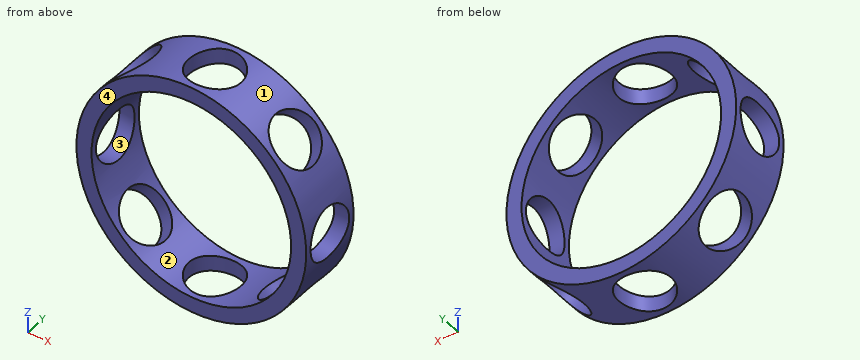
```python
from build123d import *

# Parameters (mm, degrees)
BOSS_EXTRUDE1_DEPTH      = 0.93218
BOSS_EXTRUDE1_DEPTH_BACK = 0.93218
SKETCH1_R                = 3.39852
SKETCH1_R_2              = 2.95148
CUT_EXTRUDE1_REACH       = 6.896
CUT_EXTRUDE1_END_RADIUS  = 3.39852
SKETCH3_R                = 0.762
CIRPATTERN1_COUNT        = 8


with BuildPart() as part:
    # Sketch1 → Boss-Extrude1 (new, two sides: drawn at the far end of the back side and taken through both)
    with BuildSketch(Plane(origin=(0, 0, 0), x_dir=(1, 0, 0), z_dir=(0, 1, 0)).offset(-BOSS_EXTRUDE1_DEPTH_BACK)):
        with Locations(Location((0, 0, 0), (0, 0, 270))):
            Circle(SKETCH1_R)
        with Locations(Location((0, 0, 0), (0, 0, 270))):
            Circle(SKETCH1_R_2, mode=Mode.SUBTRACT)
    extrude(amount=BOSS_EXTRUDE1_DEPTH + BOSS_EXTRUDE1_DEPTH_BACK)

    # Cut-Extrude1: up to this cylinder (the profile starts inside it)
    cut_extrude1_end = Plane(origin=(0, 0, 0), z_dir=(0, 1, 0)) * Cylinder(CUT_EXTRUDE1_END_RADIUS, 21.58904, mode=Mode.PRIVATE)
    # Sketch3 → Cut-Extrude1 (cut, up to the surface)
    with BuildSketch(Plane.XY, mode=Mode.PRIVATE) as cut_extrude1_sk1:
        Circle(SKETCH3_R)
    cut_extrude1_tool1 = extrude(cut_extrude1_sk1.sketch, amount=-CUT_EXTRUDE1_REACH, mode=Mode.PRIVATE) & cut_extrude1_end
    cut_extrude1 = cut_extrude1_tool1.solids().sort_by_distance((0, 0, 0))[0]
    add(cut_extrude1, mode=Mode.SUBTRACT)

    # CirPattern1: Cut-Extrude1 ×8 about axis
    cirpattern1_axis = Axis((0, 0, 0), (0, 1, 0))
    for i in range(1, CIRPATTERN1_COUNT):
        add(cut_extrude1.rotate(cirpattern1_axis, i * 360 / CIRPATTERN1_COUNT), mode=Mode.SUBTRACT)


solid = part.part
```
The listing builds one solid part. Answer for the finished solid, in the listing's coordinates (mm). Face numbers are marked on the shaded views. Give positions to 0.01 mm unless a question says otherwise; leave off trailing zeros. Order: outer loops, then holes, each group sorted by start corner. A loop starts at its lowest first (then second) coordinate and runs counter-clockwise, first axis right, second up. Notation, with made-up numbers: (69.25, 38.25) -> (105.25, 38.25) arc R29 cw to (105.25, 63.25) -> close; hole circle Ø11 at (81.5, 50). An arc over 180 degrees is marked (long way). Answer as CSV lines item,"result". Start each with the question number.
Q1. Determine the mould class of the marked faces 1, 2, 3 and 4 for opening direction Z: pulls with the +Z half, pulls with the -Z half, needs draft (parallel to the pull), parting line crosses it, or undercut.
Q2. Find the intervals of material crossed by L1, parallel to Y at x = 0, z = 3.05; L2, parallel to X at y = -0.4, z = -1; L3, parallel to X at y = -0.45, z = 1.25, in increasing order.
Q3. A cutting plane is placed at A-A (z = 0). Determine the outline of the cut face in (x, y).
Q4. A cutting plane is placed at B-B (y = 0). Count the separate pieces of the cut face and the enclosed holes in it, then the cut area to 3 significant figures.
Results found:
1,face 1,"parting line crosses it"
1,face 2,"undercut"
1,face 3,"undercut"
1,face 4,"needs draft"
2,L1,"-0.93 to -0.76, 0.76 to 0.93"
2,L2,"-3.25 to -2.78, 2.78 to 3.25"
2,L3,"-3.16 to -2.67, 2.67 to 3.16"
3,outline,"(-3.4, -0.93) -> (-2.95, -0.93) -> (-2.95, -0.76) -> (-3.4, -0.76) -> close; (-3.4, 0.76) -> (-2.95, 0.76) -> (-2.95, 0.93) -> (-3.4, 0.93) -> close; (2.95, -0.93) -> (3.4, -0.93) -> (3.4, -0.76) -> (2.95, -0.76) -> close; (2.95, 0.76) -> (3.4, 0.76) -> (3.4, 0.93) -> (2.95, 0.93) -> close"
4,separate pieces,"8"
4,enclosed holes,"0"
4,area,"3.41 mm2"
